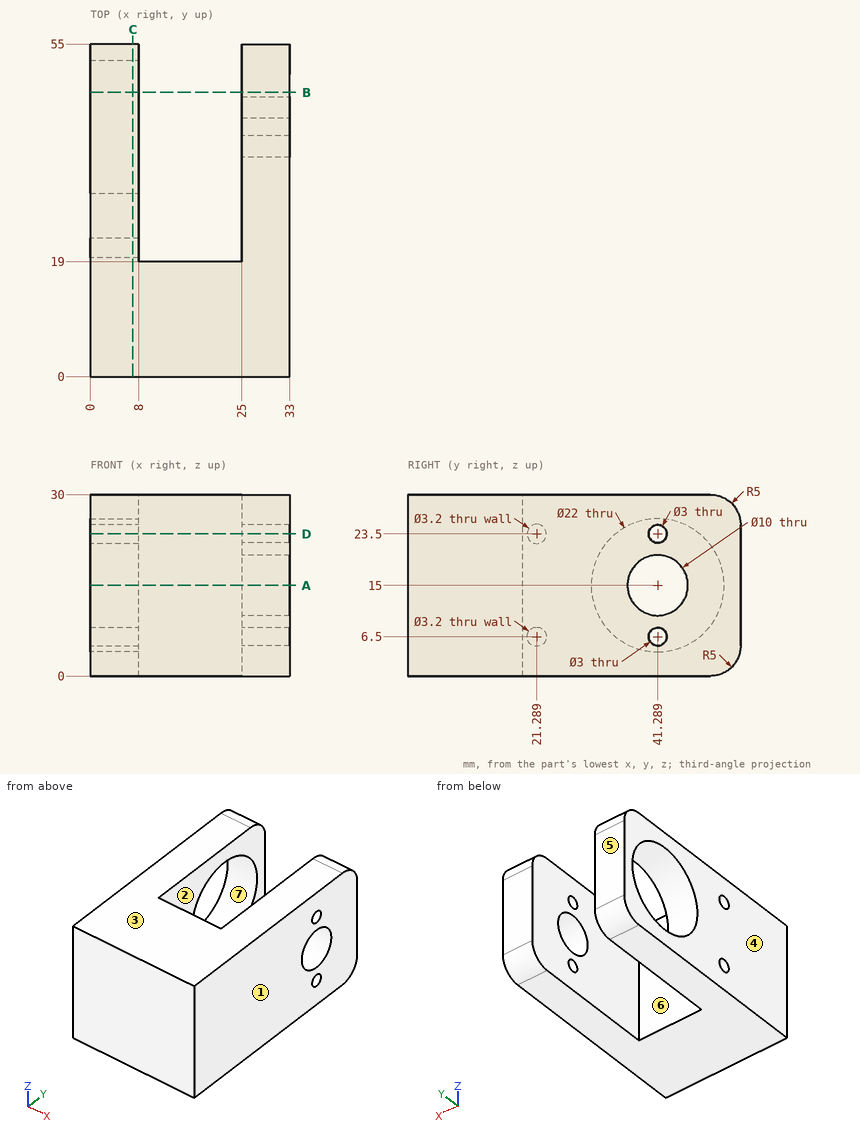
Part print with two shaded views. Sizes in mm from the minimum x, y, z corner. A direction names the side the tool comes from. Coordinates: 2 decimals unless noted, no trailing zeros. Write each loop counter-clockwise with the first axis right and the second up, starting at its lowest first coordinate (ties: lowest second). Pieces come first, ordered by that corner, then holes.
1. Band-saw the part on A-A, the plane z = 15. Give the cut face in (x, y).
Answer block:
outline: (0, 0) - (33, 0) - (33, 36.29) - (25, 36.29) - (25, 19) - (8, 19) - (8, 30.29) - (0, 30.29) - close; (0, 52.29) - (8, 52.29) - (8, 55) - (0, 55) - close; (25, 46.29) - (33, 46.29) - (33, 55) - (25, 55) - close
2. Band-saw the part on B-B, the plane y = 47. Give the cut face in (x, z).
Answer block:
outline: (0, 0) - (8, 0) - (8, 5.6) - (0, 5.6) - close; (0, 24.4) - (8, 24.4) - (8, 30) - (0, 30) - close; (25, 0) - (33, 0) - (33, 30) - (25, 30) - close
3. Band-saw the part on C-C, the plane x = 7. Give the cut face in (y, z).
Answer block:
outline: (0, 0) - (50, 0) arc R5 ccw to (55, 5) - (55, 25) arc R5 ccw to (50, 30) - (0, 30) - close; hole circle Ø3.2 at (21.29, 6.5); hole circle Ø3.2 at (21.29, 23.5); hole circle Ø22 at (41.29, 15)
4. Pull direction X, two halves, no side cores. Call the marked faces 1, 2, 3 and 4: released by +X, released by -X, zero draft, split by the parting line, or undercut.
Answer block:
face 1: released by +X
face 2: undercut
face 3: zero draft
face 4: released by -X
5. Drop flat-ended pins along their axis: pin 1 (5 mm diameter, centred on x = 24, z = 6.5, fed in from +Y); pin 2 (1 mm diameter, centred on y = 45, z = 23.5, fed in from -X); pin 3 (3 mm diameter, centred on x = 21, z = 25, fed in from +Y). Give the stop position or say it passes through.
Answer block:
pin 1: stops at y = 55
pin 2: stops at x = 25
pin 3: stops at y = 19
6. Drill centre lines: probe 1 along X at (y, z) = (29, 17); probe 2 along Y at (x, z) = (29.25, 6.5); probe 3 along Y at (x, z) = (3, 23.5) (1 decimal). Where is each one in solid material? Low to high.
Answer block:
probe 1: x = 0 to 8, 25 to 33
probe 2: y = 0 to 39.79, 42.79 to 55
probe 3: y = 0 to 19.7, 22.9 to 34.3, 48.3 to 55
7. Band-saw the part on D-D, the plane z = 23.5. Give the cut face in (x, y).
Answer block:
outline: (0, 0) - (33, 0) - (33, 39.79) - (25, 39.79) - (25, 19) - (8, 19) - (8, 19.69) - (0, 19.69) - close; (0, 22.89) - (8, 22.89) - (8, 34.31) - (0, 34.31) - close; (0, 48.27) - (8, 48.27) - (8, 55) - (0, 55) - close; (25, 42.79) - (33, 42.79) - (33, 55) - (25, 55) - close
8. 3-axis set-ups, long thin cutter, end or side, ignore diameter. For the marked faces 5, 6 and 7: which of +Z, -Z, +X, -X, +Y, -Y reach the whole face in a straight line?
Answer block:
face 5: +Z, -Z, +X, -X, +Y
face 6: +Z, -Z, +Y
face 7: -X
